Geometry: final body of the model. Coordinates: model frame, mm. A direction names the side the tool comes from. Round coordinates to 2 decimals unless told otherwise and drop trailing zeros. Order: outer loops, then holes, each group sorted by start corner. A loop starts at its lowest first (then second) coordinate and runs counter-clockwise, first axis right, second up. Notation, with made-up numbers: (81, 44.5) -> (98, 44.5) arc R27 ccw to (98, 66.5) -> close; hole circle Ø9 at (21.5, 41.5). An arc over 180 degrees is marked (long way). Put each result on its own line as item: value.
```python
from build123d import *

# Parameters (mm, degrees)
LOX_INSTALL_SIZE    = 1.5875
O_RING_INSTALL_SIZE = 1.5875


with BuildPart() as part:
    # Sketch1 → Revolve1 (revolve)
    with BuildSketch(Plane.XY, mode=Mode.PRIVATE) as revolve1_sk:
        Polygon((0, 0), (24.13, 0), (24.13, -6.35), (25.4, -6.35), (25.4, -13.97), (24.13, -13.97), (24.13, -19.05), (0, -19.05), align=None)
    revolve(revolve1_sk.sketch.rotate(Axis((0, 0, 0), (0, -1, 0)), 90), axis=Axis((0, 0, 0), (0, -1, 0)))

    # lox install
    lox_install_edges = [part.edges().sort_by_distance(p)[0] for p in [
        (0, 0, -24.13),
    ]]
    chamfer(lox_install_edges, length=LOX_INSTALL_SIZE)

    # o-ring install
    o_ring_install_edges = [part.edges().sort_by_distance(p)[0] for p in [
        (0, -19.05, -24.13),
    ]]
    chamfer(o_ring_install_edges, length=O_RING_INSTALL_SIZE)


solid = part.part
```
1. Cut plane D-D on y = -8. Return loops of the section in (x, z).
Ans:
outline: circle Ø50.8 at (0, 0)
2. Cut plane C-C on y = -2.25. Return loops of the section in (x, z).
Ans:
outline: circle Ø48.26 at (0, 0)
3. Material intervals for probe 1 along Y at (x, z) = (-12, 22); probe 2 along X at (y, z) = (-3.25, 4.5); probe 3 along Y at (x, z) = (15, 17.5), sorted ascending.
Ans:
probe 1: -13.97 to -6.35
probe 2: -23.71 to 23.71
probe 3: -18.54 to -0.51
4. Cut plane B-B on z = 0. Return loops of the section in (x, y).
Ans:
outline: (-25.4, -13.97) -> (-24.13, -13.97) -> (-24.13, -17.46) -> (-22.54, -19.05) -> (22.54, -19.05) -> (24.13, -17.46) -> (24.13, -13.97) -> (25.4, -13.97) -> (25.4, -6.35) -> (24.13, -6.35) -> (24.13, -1.59) -> (22.54, 0) -> (-22.54, 0) -> (-24.13, -1.59) -> (-24.13, -6.35) -> (-25.4, -6.35) -> close
5. Set-up query: faces 1 (the face through (-7.248, -4.002, 23.016)), 2 (the face through (0, -19.05, 0)), 3 (the face through (-7.248, -15.741, 23.016)). Return all of +Z, -Z, +X, -X, +Y, -Y with unobstructed straight access to the full face (end or side cutting, diameter ignored); none if empty.
Ans:
face 1: +Y
face 2: +Z, -Z, +X, -X, -Y
face 3: -Y
6. Cut plane A-A on x = 0. Return loops of the section in (y, z), and give its area (3 significant figures).
Ans:
outline: (-19.05, -22.54) -> (-17.46, -24.13) -> (-13.97, -24.13) -> (-13.97, -25.4) -> (-6.35, -25.4) -> (-6.35, -24.13) -> (-1.59, -24.13) -> (0, -22.54) -> (0, 22.54) -> (-1.59, 24.13) -> (-6.35, 24.13) -> (-6.35, 25.4) -> (-13.97, 25.4) -> (-13.97, 24.13) -> (-17.46, 24.13) -> (-19.05, 22.54) -> close
area: 934 mm²
7. Contact query for flat-ended pins moving along their axis: P1, Ø10, axis at y = -7, z = 12.5, coming from the +X side; P2, Ø2, axis at x = 4, y = -7, coming from the -Z side; P3, Ø2, axis at y = -9.5, z = 3.5, coming from the +X side; P4, Ø4, axis at x = 1.5, z = 0.5, coming from the +Y side. Output: stop coordinate, or through.
Ans:
P1: x = 24.27
P2: z = -25.22
P3: x = 25.28
P4: y = 0
